For this review, take the finished solid that the model builds, in its own axes (mm). Round coordinates to 2 decimals unless told otherwise and drop trailing zeros. Loops run counter-clockwise (first coordinate to the right, second up) from the corner with the lowest first, then second, coordinate; pieces in that order, holes last.
1) Mouldability with a two-part tool opening along Y and no side actions: class faces 1 (the cylindrical face through (4.84, 37.59, 30.42)), 2 (the flat face through (32.79, 19.234, 29.65)), 3 (the flat face through (13, 28, 60)) as pulls with the +Y half, pulls with the -Y half, needs draft (parallel to the pull), parting line crosses it, or undercut.
2) Take a section at A-A (z = 47). State the section outline as (x, y) points.
3) Insertion check: pin 1 (16 mm diameter, centred on x = 0, y = 30, fed in from +Z); pin 2 (3 mm diameter, centred on y = 32.5, z = 30, fed in from -X); pin 3 (5 mm diameter, centred on x = 24.5, z = 28, fed in from -Y) (3 decimals); pin 4 (2 mm diameter, centred on x = 44.5, z = 28, fed in from -Y). Each pin has a flat end and moves straight along its axis. Give the tip position at first contact, or say it passes through.
4) Wall thickness on L1, parallel to Y at x = 0, z = 39; L2, parallel to X at y = 27, z = 3; L3, parallel to Y at x = -17.5, z = 8.5: over which ranges is each line inside the solid? List them lowest first.
```python
from build123d import *

# Parameters (mm, degrees)
F1_DEPTH = 60
F2_R     = 9
F3_DEPTH = 60.001
F4_R     = 5
F5_R     = 5


with BuildPart() as f1:
    # F0 (on Top) → F1 (new body)
    with BuildSketch(Plane.XY):
        Polygon((-45.866266, 46.307288), (0, 0), (78.942902, 46.307288), align=None)
    extrude(amount=F1_DEPTH)

    # F2 (on face) → F3 (cut, through all)
    with BuildSketch(Plane.XY.offset(60)):
        with Locations((0, 30)):
            Circle(F2_R)
    extrude(amount=-F3_DEPTH, mode=Mode.SUBTRACT)

    # F4
    f4_edges = [f1.edges().sort_by_distance(p)[0] for p in [
        (-45.866266, 46.307288, 30),
        (0, 0, 30),
        (78.942902, 46.307288, 30),
    ]]
    fillet(f4_edges, radius=F4_R)

    # F5
    f5_edges = [f1.edges().sort_by_distance(p)[0] for p in [
        (33.208191, 19.479665, 0),
        (33.208191, 19.479665, 60),
    ]]
    fillet(f5_edges, radius=F5_R)


solid = f1.part
```
Response:
1. face 1: undercut
1. face 2: pulls with the -Y half
1. face 3: needs draft
2. outline: (-37.43, 37.79) - (-2.73, 2.76) arc R5 ccw to (3.35, 1.96) - (63.07, 36.99) arc R5 ccw to (60.54, 46.31) - (-33.88, 46.31) arc R5 ccw to start; hole circle Ø18 at (0, 30)
3. pin 1: passes through
3. pin 2: stops at x = -33.68
3. pin 3: stops at y = 12.905
3. pin 4: stops at y = 25.52
4. L1: y = 1.35 to 21, 39 to 46.31
4. L2: x = -26.16 to -8.49, 8.49 to 45.2
4. L3: y = 17.67 to 46.31
